```python
from build123d import *

# Parameters (mm, degrees)
SKETCH_1_R             = 5.4
EXTRUDE_1_DEPTH        = 60
CHAMFER_1_SIZE         = 0.5
SKETCH_2_R             = 4
EXTRUDE_2_DEPTH        = 8
CHAMFER_2_SIZE         = 0.5
HOLE_WIZARD_M5_1_D     = 4.2
HOLE_WIZARD_M5_1_DEPTH = 12.4
HOLE_WIZARD_M5_1_TIP   = 1.2618073
CHAMFER_3_SIZE         = 0.5
SKETCH_5_W             = 10
SKETCH_5_H             = 3
CUT_EXTRUDE_3_DEPTH    = 13
CHAMFER_4_SIZE         = 0.5


with BuildPart() as part:
    # 草图1 → 拉伸1 (new body)
    with BuildSketch(Plane.XY):
        Circle(SKETCH_1_R)
    extrude(amount=EXTRUDE_1_DEPTH)

    # 倒角1
    chamfer_1_edges = [part.edges().sort_by_distance(p)[0] for p in [
        (-5.4, 0, 0),
        (-5.4, 0, 60),
    ]]
    chamfer(chamfer_1_edges, length=CHAMFER_1_SIZE)

    # 草图2 → 拉伸2 (add)
    with BuildSketch(Plane.XY.offset(60)):
        Circle(SKETCH_2_R)
    extrude(amount=EXTRUDE_2_DEPTH)

    # 倒角2
    chamfer_2_edges = [part.edges().sort_by_distance(p)[0] for p in [
        (-4, 0, 68),
    ]]
    chamfer(chamfer_2_edges, length=CHAMFER_2_SIZE)

    # M5 螺纹孔1
    with Locations(Plane(origin=(0, 0, 0), x_dir=(-1, 0, 0), z_dir=(0, 0, -1))):
        with Locations((0, 0)):
            Hole(HOLE_WIZARD_M5_1_D / 2, depth=HOLE_WIZARD_M5_1_DEPTH)
            with Locations((0, 0, -(HOLE_WIZARD_M5_1_DEPTH + HOLE_WIZARD_M5_1_TIP / 2))):  # 118° drill point
                Cone(0, HOLE_WIZARD_M5_1_D / 2, HOLE_WIZARD_M5_1_TIP, mode=Mode.SUBTRACT)

    # 倒角3
    chamfer_3_edges = [part.edges().sort_by_distance(p)[0] for p in [
        (-2.1, 0, 0),
    ]]
    chamfer(chamfer_3_edges, length=CHAMFER_3_SIZE)

    # 草图5 → 拉伸3 (cut)
    with BuildSketch(Plane.XY):
        with Locations((0, 6.5)):
            Rectangle(SKETCH_5_W, SKETCH_5_H)
    cut_extrude_3 = extrude(amount=CUT_EXTRUDE_3_DEPTH, mode=Mode.SUBTRACT)

    # 镜向1: 拉伸3 across plane
    add(cut_extrude_3.mirror(Plane.ZX), mode=Mode.SUBTRACT)

    # 倒角4
    chamfer_4_edges = [part.edges().sort_by_distance(p)[0] for p in [
        (-4, 0, 60),
    ]]
    chamfer(chamfer_4_edges, length=CHAMFER_4_SIZE)


solid = part.part
```
The model under review builds one solid part; all positions refer to its coordinate system, in mm. A direction names the side the tool comes from. Give positions to 0.01 mm unless a question says otherwise; leave off trailing zeros. Write each loop counter-clockwise with the first axis right and the second up, starting at its lowest first coordinate (ties: lowest second). Pieces come first, ordered by that corner, then holes.
(1) For P1, Ø1.5, axis at y = -2, z = 37, coming from the -X side; P2, Ø1, axis at x = 0.5, z = 56, coming from the +Y side; P3, Ø3.5, axis at x = 0, z = 6.5, coming from the -Y side; P4, Ø3.5, axis at x = 0, z = 6, coming from the +Y side, all flat-tipped, find the tip position at first contact; note any pin that passes through.
(2) To check wall thickness, follow L1, parallel to X at y = 0, z = 4.75; L2, parallel to Y at x = 0, z = 5; L3, parallel to Y at x = -0.5, z = 10. State the ranges of each line that lie inside material, in increasing order.
(3) The part is to be moulded in two halves that separate along Y. For faces 4 (the flat face through (0, 5, 6)), 5 (the cylindrical face through (2.003, 0.631, 6.533)), 6 (the conical face through (-0.35, 0.11, 13.44)), 7 (the cylindrical face through (5.15, 1.62, 29.59)), say which applies: released by +Y, released by -Y, zero draft, split by the parting line, or undercut.
(4) Consider section A-A, the plane z = 48. Give the boundary of the cut face in (x, y), and give its area (3 significant figures).
(5) Consider section B-B, the plane z = 63.5. Give the boundary of the cut face in (x, y), and give its area (3 significant figures).
(6) Tool access review of faces 1 (the flat face through (0, -5, 6)), 2 (the cylindrical face through (-0.867, -3.905, 63.951)), 3 (the flat face through (0, 0, 68)): name each direction out of +Z, -Z, +X, -X, +Y, -Y from which nothing blocks a thin tool from reaching the whole face with its end or side.
Returned:
1. P1: stops at x = -5.25
1. P2: stops at y = 5.4
1. P3: stops at y = -5
1. P4: stops at y = 5
2. L1: x = -5.4 to -2.1, 2.1 to 5.4
2. L2: y = -5 to -2.1, 2.1 to 5
2. L3: y = -5 to -2.04, 2.04 to 5
3. face 4: released by +Y
3. face 5: undercut
3. face 6: undercut
3. face 7: split by the parting line
4. outline: circle Ø10.8 at (0, 0)
4. area: 91.6 mm2
5. outline: circle Ø8 at (0, 0)
5. area: 50.3 mm2
6. face 1: -Z, +X, -X, -Y
6. face 2: +Z
6. face 3: +Z, +X, -X, +Y, -Y
